Build history of the part. All positions in model axes, mm. Round coordinates to 2 decimals unless told otherwise and drop trailing zeros. Loops run counter-clockwise (first coordinate to the right, second up) from the corner with the lowest first, then second, coordinate; pieces in that order, holes last. Notation, with made-up numbers: (80.5, 89) - (138.5, 89) arc R25 ccw to (138.5, 107) - close; hole circle Ø9 at (22.5, 74.5). An arc over 180 degrees is marked (long way). Use a Markdown table: item, result.
from build123d import *

# Parameters (mm, degrees)
F1_R     = 12
F1_R_2   = 10
F2_DEPTH = 4
F5_DEPTH = 4


# Not quite as in the source:
# - a fillet or chamfer that OpenCascade refuses, or shapes differently, is made with other operations: its cross-section is extruded or revolved along the edge and cut away or added


with BuildPart() as f2:
    # F1 (on Front) → F2 (new body)
    with BuildSketch(Plane.XZ):
        Circle(F1_R)
        Circle(F1_R_2, mode=Mode.SUBTRACT)
    extrude(amount=F2_DEPTH)

    # F3: fillet of radius 5 on 1 edges, made by hand

    # F3_s1 → F3_t2 (revolve, cut)
    with BuildSketch(Plane.XY):
        with BuildLine():
            ThreePointArc((10, -4), (10.527864045, -1.7639320225), (12, 0))
            Line((12, 0), (10, 0))
            Line((10, 0), (10, -4))
        make_face()
    revolve(axis=Axis((0, 0, 0), (0, -1, 0)), mode=Mode.SUBTRACT)

    # F4 (on face) → F5 (join)
    with BuildSketch(Plane.XZ.offset(4)):
        with BuildLine():
            ThreePointArc((-11.8377969718, 1.9663577638), (-11.6917562913, 2.7023757741), (-11.5, 3.4278273002))
            ThreePointArc((-11.5, 3.4278273002), (-19.0279514026, 0), (-11.5, -3.4278273002))
            ThreePointArc((-11.5, -3.4278273002), (-11.6917562913, -2.7023757741), (-11.8377969718, -1.9663577638))
            ThreePointArc((-11.8377969718, -1.9663577638), (-17.78, 0), (-11.8377969718, 1.9663577638))
        make_face()
    extrude(amount=-F5_DEPTH)


solid = f2.part
Q1. Probe line 1 (X direction, y = -3.3, z = -3.75); line 2 (X direction, y = -2.95, z = -1.5); line 3 (Z direction, x = -1.5, y = -0.65). List the from-to ranges inside material, lowest first.
Results found:
| item | result |
|---|---|
| line 1 | x = -17.05 to -11.92, -11.4 to -9.32, 9.32 to 11.4 |
| line 2 | x = -18.77 to -17.42, -11.91 to -10, 10 to 11.91 |
| line 3 | z = -11.91 to -11.19, 11.19 to 11.91 |
Q2. Cut at C-C, the plane y = -0.6. List the corners of the cut face in (x, z).
Results found:
| item | result |
|---|---|
| outline | (-11.5, -3.43) arc R12 ccw (long way) to (-11.5, 3.43) arc R4.54 ccw (long way) to start; hole (-11.84, -1.97) arc R12 cw to (-11.84, 1.97) arc R3.3 ccw (long way) to start; hole circle Ø22.67 at (0, 0) |
Q3. Drop flat-ended pins along their axis: pin 1 (5 mm diameter, centred on x = -6, z = 2, fed in from -Y); pin 2 (1.5 mm diameter, centred on x = -1, y = -1.5, fed in from -Z); pin 3 (1 mm diameter, centred on x = 5, y = -0.5, fed in from -Z). Give the stop position or say it passes through.
Results found:
| item | result |
|---|---|
| pin 1 | passes through |
| pin 2 | stops at z = -12 |
| pin 3 | stops at z = -11.12 |
Q4. Pull direction X, two halves, no side cores. Call faces 1 (the face through (-12, -2, 0)), 2 (the face through (-9, -4, 5)): pulls with the +X half, pulls with the -X half, needs draft (parallel to the pull), parting line crosses it, or undercut.
Results found:
| item | result |
|---|---|
| face 1 | undercut |
| face 2 | needs draft |
Q5. Cut at B-B, the plane x = -13. List the corners of the cut face in (y, z).
Results found:
| item | result |
|---|---|
| outline | (-4, -4.3) - (0, -4.3) - (0, -2.94) - (-4, -2.94) - close; (-4, 2.94) - (0, 2.94) - (0, 4.3) - (-4, 4.3) - close |
Q6. Cut at D-D, the plane x = 0. List the corners of the cut face in (y, z).
Results found:
| item | result |
|---|---|
| outline | (-4, -12) - (0, -12) arc R5 ccw to (-4, -10) - close; (-4, 10) arc R5 ccw to (0, 12) - (-4, 12) - close |
Q7. Cut at A-A, the plane z = 0. List the corners of the cut face in (x, y), plus the area to 3 significant figures.
Results found:
| item | result |
|---|---|
| outline | (-19.03, -4) - (-17.78, -4) - (-17.78, 0) - (-19.03, 0) - close; (-12, -4) - (-10, -4) arc R5 ccw to (-12, 0) - close; (10, -4) - (12, -4) - (12, 0) arc R5 ccw to start |
| area | 16.2 mm2 |
